Could you check a few things on this model? Use its own coordinates, in mm. Give positions to 0.01 mm unless a question says otherwise; leave off trailing zeros. Loops run counter-clockwise (first coordinate to the right, second up) from the corner with the lowest first, then second, coordinate; pieces in that order, holes last. Notation, with made-up numbers: (12.25, -4) -> (29.25, -4) arc R24 ccw to (29.25, 7) -> close; hole circle Ø3 at (73.25, 82.25). An arc over 180 degrees is marked (long way). Write each question's results on one line, items separated by ' | '. Start each with the question number.
Q1. We'd pull the mould along Z, two halves only. Please class faces 1 (the face through (5, 12, 37.9)), 2 (the face through (5, 11, -15.4)), 3 (the face through (4.93, 0.774, 1.468)): released by +Z, released by -Z, zero draft, split by the parting line, or undercut.
Q2. Will this pin go through, and if not, where does the flat tip stop? P1, Ø3, axis at y = 23.5, z = 15, coming from the -X side.
Q3. If we section it at B-B, the plane y = 18.75: List the corners of the cut face in (x, z) for me.
Q4. If I drill on line 1 along Z through (x, y) = (3.25, 18.75); line 2 along Z through (x, y) = (7.75, 2.5); line 3 along Y through (x, z) = (6.75, 18), over which ranges is the centre line in solid material (lowest first)?
Q5. If we section it at A-A, the plane z = 3.75: List the corners of the cut face in (x, y) for me, plus the area to 3 significant figures.
Q6. If we section it at C-C, the plane x = 3.75: List the corners of the cut face in (y, z) for me, plus the area to 3 significant figures.
from build123d import *

# Parameters (mm, degrees)
F0_R     = 3.75
F0_W     = 11.25
F0_H     = 30.8000000767
F0_W_2   = 11.2448162399
F0_H_2   = 30.8000003636
F1_DEPTH = 10


# Not quite as in the source:
# - ends of sketch curves that miss each other by under 0.0002 mm in the source are joined


with BuildPart() as f1:
    # F0 (on Right) → F1 (new body)
    with BuildSketch(Plane.YZ):
        Polygon((11.25, 26.6500003636), (-4.1499999352, 26.6500003636), (-4.1499999352, -4.15), (11.25, -4.15), (26.65, -4.15), (26.65, 26.65), align=None)
        with Locations((3.75, 3.75)):
            Circle(F0_R, mode=Mode.SUBTRACT)
        with Locations((18.75, 3.75)):
            Circle(F0_R, mode=Mode.SUBTRACT)
        with Locations((3.75, 18.75)):
            Circle(F0_R, mode=Mode.SUBTRACT)
        with Locations((18.75, 18.75)):
            Circle(F0_R, mode=Mode.SUBTRACT)
        with Locations((32.275, 11.2500000384)):
            Rectangle(F0_W, F0_H)
        Polygon((11.25, -4.15), (-4.1499999352, -4.15), (-15.3948161751, -4.15), (-15.3948161751, -15.4), (-4.1499999352, -15.4), (26.65, -15.4), (37.9, -15.4), (37.9, -4.15), (26.65, -4.15), align=None)
        Polygon((-15.3948161751, 26.6500003636), (-4.1499999352, 26.6500002869), (11.25, 26.6500003636), (26.65, 26.65), (37.9, 26.65), (37.9000000767, 37.9), (-15.3948160984, 37.9000003636), align=None)
        with Locations((-9.7724080551, 11.2500001818)):
            Rectangle(F0_W_2, F0_H_2)
    extrude(amount=F1_DEPTH)


solid = f1.part
Final values:
1) face 1: released by +Z | face 2: released by -Z | face 3: undercut
2) P1: stops at x = 0
3) outline: (0, -15.4) -> (10, -15.4) -> (10, 0) -> (0, 0) -> close; (0, 7.5) -> (10, 7.5) -> (10, 15) -> (0, 15) -> close; (0, 22.5) -> (10, 22.5) -> (10, 37.9) -> (0, 37.9) -> close
4) line 1: z = -15.4 to 0, 7.5 to 15, 22.5 to 37.9 | line 2: z = -15.4 to 0.21, 7.29 to 15.21, 22.29 to 37.9 | line 3: y = -15.39 to 0.08, 7.42 to 15.08, 22.42 to 37.9
5) outline: (0, -15.39) -> (10, -15.39) -> (10, 0) -> (0, 0) -> close; (0, 7.5) -> (10, 7.5) -> (10, 15) -> (0, 15) -> close; (0, 22.5) -> (10, 22.5) -> (10, 37.9) -> (0, 37.9) -> close | area: 383 mm²
6) outline: (-15.39, -15.4) -> (37.9, -15.4) -> (37.9, 37.9) -> (-15.39, 37.9) -> close; hole circle Ø7.5 at (3.75, 3.75); hole circle Ø7.5 at (3.75, 18.75); hole circle Ø7.5 at (18.75, 3.75); hole circle Ø7.5 at (18.75, 18.75) | area: 2,660 mm²
